from build123d import *

# Parameters (mm, degrees)
BOSS_EXTRUDE1_DEPTH = 3.175
SKETCH2_R           = 3.175
CUT_EXTRUDE1_DEPTH  = 67.929307933


with BuildPart() as part:
    # Sketch1 → Boss-Extrude1 (new body)
    with BuildSketch(Plane.XY):
        with BuildLine():
            Line((-28.328951223, 3.070773738), (-28.328951223, -34.922456704))
            Line((-28.328951223, -34.922456704), (-28.328951223, -57.147456704))
            ThreePointArc((-28.328951223, -57.147456704), (-27.399015253, -59.392520734), (-25.153951223, -60.322456704))
            Line((-25.153951223, -60.322456704), (25.646048777, -60.322456704))
            ThreePointArc((25.646048777, -60.322456704), (27.891112807, -59.392520734), (28.821048777, -57.147456704))
            Line((28.821048777, -57.147456704), (28.821048777, -34.922456704))
            Line((28.821048777, -34.922456704), (28.821048777, 3.070773738))
            ThreePointArc((28.821048777, 3.070773738), (27.891112807, 5.315837768), (25.646048777, 6.245773738))
            Line((25.646048777, 6.245773738), (-25.153951223, 6.245773738))
            ThreePointArc((-25.153951223, 6.245773738), (-27.399015253, 5.315837768), (-28.328951223, 3.070773738))
        make_face()
    extrude(amount=-BOSS_EXTRUDE1_DEPTH)

    # Sketch2 → Cut-Extrude1 (cut, through all)
    with BuildSketch(Plane.XY):
        with Locations((-17.152951223, -5.184226262)):
            Circle(SKETCH2_R)
        with Locations(Location((17.645048777, -5.184226262, 0), (0, 0, 180))):
            Circle(SKETCH2_R)
    extrude(amount=-CUT_EXTRUDE1_DEPTH, mode=Mode.SUBTRACT)


solid = part.part
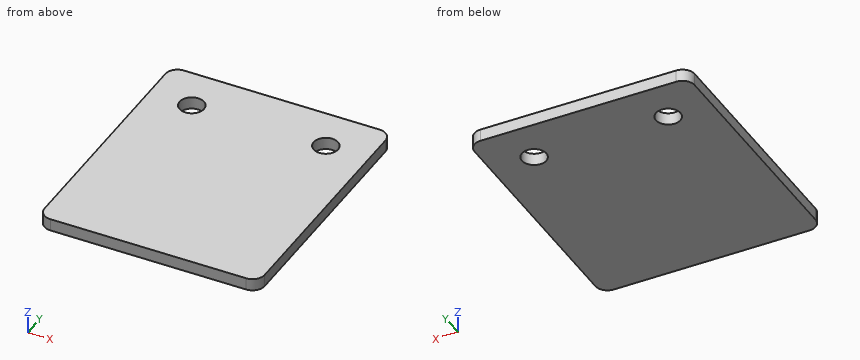
CAD build for the part. Positions are in the model's coordinates, mm. Give positions to 0.01 mm unless a question says otherwise; leave off trailing zeros. Write each loop counter-clockwise with the first axis right and the second up, starting at its lowest first coordinate (ties: lowest second). Pieces come first, ordered by that corner, then holes. Notation, with made-up numbers: (31, -6) - (88, -6) arc R26 cw to (88, 27) - close; hole circle Ø10 at (-25, 69). An arc over 180 degrees is marked (long way). Put each result on its own line as item: value.
(1) Saw through at B-B (z = -1). List the corners of the cut face in (x, y) (3 decimals).
Working result:
outline: (-28.329, -57.147) arc R3.175 ccw to (-25.154, -60.322) - (25.646, -60.322) arc R3.175 ccw to (28.821, -57.147) - (28.821, 3.071) arc R3.175 ccw to (25.646, 6.246) - (-25.154, 6.246) arc R3.175 ccw to (-28.329, 3.071) - close; hole circle Ø6.35 at (-17.153, -5.184); hole circle Ø6.35 at (17.645, -5.184)
(2) Saw through at A-A (y = -4). List the corners of the cut face in (x, z) (3 decimals), then the cut area to 3 significant figures.
Working result:
outline: (-28.329, -3.175) - (-20.099, -3.175) - (-20.099, 0) - (-28.329, 0) - close; (-14.207, -3.175) - (14.699, -3.175) - (14.699, 0) - (-14.207, 0) - close; (20.591, -3.175) - (28.821, -3.175) - (28.821, 0) - (20.591, 0) - close
area: 144 mm^2
(3) Wall check: L1, parallel to X at y = -5, z = -1.95; L2, parallel to Y at x = 19.5, z = -1.9; L3, parallel to Y at x = 18.5, z = -0.5. Give the ranges that are in metal, low to high.
Working result:
L1: -28.33 to -20.32, -13.98 to 14.48, 20.81 to 28.82
L2: -60.32 to -7.76, -2.61 to 6.25
L3: -60.32 to -8.24, -2.13 to 6.25
